Check sheet for the modelled part. Datum: model origin and axes. Units: mm. A direction names the side the tool comes from. Round coordinates to 2 decimals unless told otherwise and drop trailing zeros. Order: outer loops, then holes, each group sorted by start corner. A loop starts at its lowest first (then second) coordinate and runs counter-clockwise, first axis right, second up.
Q1. Scan lines: probe 1 along X at (y, z) = (72, 27); probe 2 along Z at (x, y) = (24.5, 80.5); probe 3 along Z at (x, y) = (47.5, 47.5). Record each from-to range of solid material in increasing order.
Q2. Cross-section at A-A on x = 28. Record the cut outline in (y, z).
Q3. Set-up check for faces 4 (the cylindrical face through (54.65, -47.701, -2.042)), 5 (the flat face through (54, -76, 0)), 6 (the flat face through (55, 65.775, 30)): record each of +Z, -Z, +X, -X, +Y, -Y from which the full face is reachable in a straight line by a thin tool's end or side.
Q4. Cross-section at C-C on y = -38. Record the cut outline in (x, z).
Q5. Depth check by flat-ended pin: P1, Ø13.5, axis at x = 63.5, y = -78, coming from the -Z side; P2, Ø4, axis at x = 88.5, y = 45.5, coming from the +Z side; P3, Ø12, axis at x = 59.5, y = 12, coming from the +Z side. Enter the tip coordinate at first touch or a pass-through.
Q6. Cross-section at D-D on z = 40.5. Record the cut outline in (x, y).
Q7. Mould release check, pull along X, two halves, no side actions. Record for faces 1 (the flat face through (54.93, 63.36, 25.17)), 2 (the flat face through (54.3, 98.47, 39.13)), 3 (the flat face through (107.535, 95.975, 38.628)): +X half, -X half, draft (parallel to the pull), parting line (faces both ways), or undercut.
Q8. Cross-section at B-B on x = 70.5. Record the cut outline in (y, z).
from build123d import *

# Parameters (mm, degrees)
F1_R         = 1.6
F2_DEPTH     = 110
F3_W         = 15
F3_H         = 15
F4_DEPTH     = 10.5
F5_R         = 1.6
F6_DEPTH     = 15
F7_T1_DEPTH  = 15
F9_DEPTH     = 5
F10_R        = 1.6
F11_DEPTH    = 110.001
F12_SIZE     = 5
F13_SIZE     = 5
F14_SIZE     = 5
F15_R        = 1.6
F16_DEPTH    = 15
F17_T1_DEPTH = 15


# Not quite as in the source:
# - a fillet or chamfer that OpenCascade refuses, or shapes differently, is made with other operations: its cross-section is extruded or revolved along the edge and cut away or added
# - an extrude ends at something that could not be found from the text; its depth is read off the source's solid


with BuildPart() as f2:
    # F1 (on Right) → F2 (new body)
    with BuildSketch(Plane.YZ):
        with BuildLine():
            Line((-97.5568636432, 0), (-53.34897794, 0))
            ThreePointArc((-53.34897794, 0), (-47.6134207396, -2.0300236301), (-42.7112703662, 1.5736597709))
            Line((-42.7112703662, 1.5736597709), (101.0891949998, 30.1261963412))
            Line((101.0891949998, 30.1261963412), (95.775378419, 48.3873994959))
            Line((95.775378419, 48.3873994959), (-97.5568636432, 10))
            Line((-97.5568636432, 10), (-97.5568636432, 0))
        make_face()
        with Locations((-48.5646284544, 3.8089532984)):
            Circle(F1_R, mode=Mode.SUBTRACT)
    extrude(amount=F2_DEPTH)

    # F3 (on Top) → F4 (cut, symmetric)
    with BuildSketch(Plane.XY):
        with Locations((22.5, -48.34897794)):
            Rectangle(F3_W, F3_H)
        with Locations((87.5, -47.7112703662)):
            Rectangle(F3_W, F3_H)
    extrude(amount=F4_DEPTH, both=True, mode=Mode.SUBTRACT)

    # F5 (on face) → F6 (cut, through all)
    with BuildSketch(Plane.YZ.offset(80)):
        with BuildLine():
            Line((-28.9665386081, -1.5009464696), (-35.5646284544, 3.8089532984))
            ThreePointArc((-35.5646284544, 3.8089532984), (-48.5646284544, 16.8089532984), (-61.5646284544, 3.8089532984))
            Line((-61.5646284544, 3.8089532984), (-67.6559507847, -1.5009464696))
            Line((-67.6559507847, -1.5009464696), (-44.5721596479, -13.8469105586))
            Line((-44.5721596479, -13.8469105586), (-28.9665386081, -1.5009464696))
        make_face()
        with Locations((-48.5646284544, 3.8089532984)):
            Circle(F5_R, mode=Mode.SUBTRACT)
    extrude(amount=F6_DEPTH, mode=Mode.SUBTRACT)

    # F7: chamfer of 5 on 1 edges, made by hand

    # F7_s2 → F7_t1 (cut)
    with BuildSketch(Plane.YZ.offset(80)):
        with BuildLine():
            Line((-64.7812034248, 0.9241461465), (-61.1056580828, 6.9991937656))
            Line((-61.1056580828, 6.9991937656), (-61.0083922357, 6.9759697482))
            ThreePointArc((-61.0083922357, 6.9759697482), (-61.3651603236, 5.4078228571), (-61.4646284544, 3.8089532984))
            Line((-61.4646284544, 3.8089532984), (-61.4989183361, 3.7335730599))
            ThreePointArc((-61.4989183361, 3.7335730599), (-63.1272340331, 2.3141451142), (-64.7154933066, 0.848765908))
            Line((-64.7154933066, 0.848765908), (-64.7812034248, 0.9241461465))
        make_face()
    extrude(amount=F7_T1_DEPTH, mode=Mode.SUBTRACT)

    # F8 (on offset) → F9 (cut, symmetric)
    with BuildSketch(Plane.YZ.offset(55)):
        with BuildLine():
            Line((77.775378419, 22.0739301294), (77.775378419, 32.4073002482))
            ThreePointArc((77.775378419, 32.4073002482), (71.775378419, 38.4073002482), (65.775378419, 32.4073002482))
            Line((65.775378419, 32.4073002482), (65.775378419, 22.0739301294))
            Line((65.775378419, 22.0739301294), (77.775378419, 22.0739301294))
        make_face()
    extrude(amount=F9_DEPTH, both=True, mode=Mode.SUBTRACT)

    # F10 (on face) → F11 (cut, through all)
    with BuildSketch(Plane.YZ.offset(110)):
        with Locations((71.775378419, 32.4073002482)):
            Circle(F10_R)
    extrude(amount=-F11_DEPTH, mode=Mode.SUBTRACT)

    # F12
    f12_edges = [f2.edges().sort_by_distance(p)[0] for p in [
        (55, 77.775378, 25.497083),
    ]]
    chamfer(f12_edges, length=F12_SIZE)

    # F13
    f13_edges = [f2.edges().sort_by_distance(p)[0] for p in [
        (55, 65.775378, 23.114404),
    ]]
    chamfer(f13_edges, length=F13_SIZE)

    # F14
    f14_edges = [f2.edges().sort_by_distance(p)[0] for p in [
        (0, 98.432287, 39.256798),
        (110, 98.432287, 39.256798),
        (110, -97.556864, 5),
        (0, -97.556864, 5),
    ]]
    chamfer(f14_edges, length=F14_SIZE)

    # F15 (on face) → F16 (cut, through all)
    with BuildSketch(Plane(origin=(30, 0, 0), x_dir=(0, -1, 0), z_dir=(-1, 0, 0))):
        with BuildLine():
            Line((68.1627183007, -1.5009464696), (61.5646284544, 3.8089532984))
            ThreePointArc((61.5646284544, 3.8089532984), (48.5646284544, 16.8089532984), (35.5646284544, 3.8089532984))
            Line((35.5646284544, 3.8089532984), (29.4733061241, -1.5009464696))
            Line((29.4733061241, -1.5009464696), (52.5570972608, -13.8469105586))
            Line((52.5570972608, -13.8469105586), (68.1627183007, -1.5009464696))
        make_face()
        with Locations((48.5646284544, 3.8089532984)):
            Circle(F15_R, mode=Mode.SUBTRACT)
    extrude(amount=F16_DEPTH, mode=Mode.SUBTRACT)

    # F17: chamfer of 5 on 1 edges, made by hand

    # F17_s2 → F17_t1 (cut)
    with BuildSketch(Plane.YZ.offset(15)):
        with BuildLine():
            Line((-64.9047662945, 1.0383670147), (-61.0901119265, 7.0462123799))
            Line((-61.0901119265, 7.0462123799), (-60.9929374028, 7.0226091613))
            ThreePointArc((-60.9929374028, 7.0226091613), (-61.3621185428, 5.4319897848), (-61.4646284544, 3.8089532984))
            Line((-61.4646284544, 3.8089532984), (-61.5019329447, 3.731047759))
            ThreePointArc((-61.5019329447, 3.731047759), (-63.1921659154, 2.3708104982), (-64.8420707848, 0.9604614753))
            Line((-64.8420707848, 0.9604614753), (-64.9047662945, 1.0383670147))
        make_face()
    extrude(amount=F17_T1_DEPTH, mode=Mode.SUBTRACT)


solid = f2.part
Results found:
1. probe 1: x = 0 to 50, 60 to 110
1. probe 2: z = 26.04 to 45.35
1. probe 3: z = 19.49 to 38.8
2. outline: (-97.56, 0) - (-66.3, 0) - (-64.8, 1.21) - (-61.2, 6.88) arc R13 cw to (-35.56, 3.81) - (-34.8, 3.14) - (101.09, 30.13) - (95.78, 48.39) - (-97.56, 10) - close; hole circle Ø3.2 at (71.78, 32.41)
3. face 4: -Z, +X, -X
3. face 5: -Z, +X, -X, -Y
3. face 6: -Z
4. outline: (0, 2.51) - (15, 2.51) - (15, 11.38) - (30, 11.38) - (30, 2.51) - (80, 2.51) - (80, 11.38) - (95, 11.38) - (95, 2.51) - (110, 2.51) - (110, 21.83) - (0, 21.83) - close
5. P1: stops at z = 0
5. P2: stops at z = 38.8
5. P3: stops at z = 32.94
6. outline: (0, 56.05) - (110, 56.05) - (110, 92.86) - (105, 98.07) - (5, 98.07) - (0, 92.86) - close
7. face 1: undercut
7. face 2: draft
7. face 3: +X half
8. outline: (-97.56, 0) - (-53.35, 0) arc R6.5 ccw to (-42.71, 1.57) - (101.09, 30.13) - (95.78, 48.39) - (-97.56, 10) - close; hole circle Ø3.2 at (-48.56, 3.81); hole circle Ø3.2 at (71.78, 32.41)
